The model under review builds one solid part; all positions refer to its coordinate system, in mm. Coordinates: 2 decimals unless noted, no trailing zeros. Order: outer loops, then holes, each group sorted by start corner. A loop starts at its lowest first (then second) coordinate and runs counter-clockwise, first axis right, second up. Notation, with made-up numbers: M 69,32.5 L 109,32.5 A37 cw 109,71.5 Z; hole C 10,-32 d4. An arc over 180 degrees is marked long. Answer as CSV lines item,"result". Start each with the question number.
Q1. Consider section A-A on y = 6.25. Write out the cut boundary in (x, z).
Q2. For P1, Ø2, axis at x = 8, y = 7.5, coming from the +Z side; P2, Ø5, axis at y = 8.5, z = 13, coming from the -X side, all flat-tipped, find the tip position at first contact; note any pin that passes through.
Q3. Consider section B-B on x = -2. Write out the cut boundary in (y, z), and give its area (3 significant figures).
Q4. Consider section D-D on z = 19.5. Write out the cut boundary in (x, y), and give its area (3 significant figures).
Q5. Consider section C-C on x = 0. Write out the cut boundary in (y, z).
Q6. Wall thickness on L1, parallel to Z at x = 0, y = 6.75; L2, parallel to X at y = 7.25, z = -1; L3, parallel to Z at x = 3.5, y = 1.75: over which ranges is each line inside the solid? List them lowest first. Write a range as [from, to].
Autodesk Inventor part; units mm, degrees
ref_plane "YZ Plane" through (0, 0, 0) normal (1, 0, 0) x (0, 1, 0)
ref_plane "XZ Plane" through (0, 0, 0) normal (0, 1, 0) x (-1, 0, 0)
ref_plane "XY Plane" through (0, 0, 0) normal (0, 0, 1) x (1, 0, 0)
sketch "Sketch1" plane through (0, 0, 0) normal (0, 1, 0) x (-1, 0, 0)
  circle A0 centre (0, 0) radius 3
  arc A1 (-5, 0) -> (5, 0) centre (0, 0) ccw
  line L0 (-10.0001, 41) -> (-10, 19) construction
  line L1 (0, 0) -> (-5, 0) construction
  line L2 (-10.0001, 30) -> (-10.0001, 37)
  arc A2 (5, 0) -> (-10.0001, 37) centre (-48.1331, 0) ccw
  arc A3 (-5, 0) -> (-10.0001, 30) centre (-97.4989, 0) ccw
  line L3 (0, 0) -> (5, 0)
  arc A4 (5, 0) -> (-5, 0) centre (0, 0) ccw construction
  dimension "d0" = 6
  dimension "d1" = 2
  dimension "d2" = 10
  dimension "d3" = 30
  dimension "d4" = 5.0001
  dimension "d5" = 7
extrude "Extrusion1" add sketch "Sketch1" along normal blind 12
properties part number "Clutch"
Evaluation:
1,outline,"M -5,0 A5 ccw 5,0 A92.5 cw 10,30 L 10,37 A53.13 ccw Z; hole C 0,0 d6"
2,P1,"stops at z = 35.94"
2,P2,"stops at x = -3.95"
3,outline,"M 0,-4.58 L 12,-4.58 L 12,-2.24 L 0,-2.24 Z; M 0,2.24 L 12,2.24 L 12,17.6 L 0,17.6 Z"
3,area,"213 mm²"
4,outline,"M -1.29,0 L 7.08,0 L 7.08,12 L -1.29,12 Z"
4,area,"100 mm²"
5,outline,"M 0,-5 L 12,-5 L 12,-3 L 0,-3 Z; M 0,3 L 12,3 L 12,22.5 L 0,22.5 Z"
6,L1,"z = [-5, -3], [3, 22.5]"
6,L2,"x = [-4.9, -2.83], [2.83, 4.9]"
6,L3,"z = [-3.57, 28.83]"
